Model file for the job. Use its own axes, mm. A direction names the side the tool comes from. Round coordinates to 2 decimals unless told otherwise and drop trailing zeros. Order: outer loops, then holes, each group sorted by start corner. A loop starts at its lowest first (then second) coordinate and runs counter-clockwise, first axis right, second up. Notation, with made-up numbers: M 85,-35.75 L 112,-35.75 A22 cw 112,2.25 Z; hole C 25.25,60 d4. An arc over 180 degrees is marked long. Return JSON: item names as keys, results as strings. Group by question number.
Item 1: Probe line 1 along Y through (x, z) = (-2.25, -8.75); line 2 along X through (y, z) = (-47.5, 1). List the from-to ranges inside material, lowest first.
Item 2: Which spindle directions (+Z, -Z, +X, -X, +Y, -Y) get a long thin tool onto all of the face, cutting with end or side? Do faces 4 (the face through (5, -49, 0.5)), 5 (the face through (0, 1, 0)), 6 (the face through (-2, -99.5, -2)), 7 (the face through (-5.78, 0.49, -7.54)), 8 (the face through (-0.5, -49, -5)). Say none if no direction does.
Item 3: Pin check, flat tips, straight feed: pin 1 Ø1.5 at (x, y) = (6, -42.5) entering from +Z; pin 2 Ø2.5 at (x, y) = (-6.5, -39.5) entering from -Z; pin 3 Ø8 at (y, z) = (-83, 8.5) entering from +X. Stop position of each tip, or through.
Item 4: Slice it at A-A on y = -38. Write the cut outline in (x, z).
Item 5: Slice it at B-B on z = 2.75. Write the cut outline in (x, y), then the cut area to 3 significant figures.
Item 6: Pull direction Y, two halves, no side cores. Call faces 1 (the face through (3.2, -100.2, -10)), 2 (the face through (0, -101, 0)), 3 (the face through (-5, -49, 0.5)): pulls with the +Y half, pulls with the -Y half, needs draft (parallel to the pull), parting line crosses it, or undercut.
from build123d import *

# Parameters (mm, degrees)
EXTRUDE_1_DEPTH          = 0.5
PATTERN_CIRCULAR_1_COUNT = 2
PATTERN_CIRCULAR_1_ANGLE = 90
SKETCH_3_R               = 9.5
EXTRUDE_2_DEPTH          = 1
SKETCH_4_R               = 10.5
EXTRUDE_3_DEPTH          = 1.5


with BuildPart() as part:
    # Эскиз1 → Бобышка-Вытянуть1 (new, symmetric)
    with BuildSketch(Plane.XY):
        with BuildLine():
            Line((-8.75, 0), (8.75, 0))
            Line((8.75, 0), (8.75, -12.322967039))
            ThreePointArc((8.75, -12.322967039), (8.57806723, -12.883595848), (8.121390676, -13.251443729))
            Line((8.121390676, -13.251443729), (3.75, -15))
            Line((3.75, -15), (8.121390676, -16.748556271))
            ThreePointArc((8.121390676, -16.748556271), (8.57806723, -17.116404152), (8.75, -17.677032961))
            Line((8.75, -17.677032961), (8.75, -78.763241336))
            ThreePointArc((8.75, -78.763241336), (8.395311893, -81.402930425), (7.356408303, -83.855366249))
            Line((7.356408303, -83.855366249), (6.593591697, -85.144633751))
            ThreePointArc((6.593591697, -85.144633751), (5.554688107, -87.597069575), (5.2, -90.236758664))
            Line((5.2, -90.236758664), (5.2, -99.5))
            Line((5.2, -99.5), (-5.2, -99.5))
            Line((-5.2, -99.5), (-5.2, -90.236758664))
            ThreePointArc((-5.2, -90.236758664), (-5.554688107, -87.597069575), (-6.593591697, -85.144633751))
            Line((-6.593591697, -85.144633751), (-7.356408303, -83.855366249))
            ThreePointArc((-7.356408303, -83.855366249), (-8.395311893, -81.402930425), (-8.75, -78.763241336))
            Line((-8.75, -78.763241336), (-8.75, -17.677032961))
            ThreePointArc((-8.75, -17.677032961), (-8.57806723, -17.116404152), (-8.121390676, -16.748556271))
            Line((-8.121390676, -16.748556271), (-3.75, -15))
            Line((-3.75, -15), (-8.121390676, -13.251443729))
            ThreePointArc((-8.121390676, -13.251443729), (-8.57806723, -12.883595848), (-8.75, -12.322967039))
            Line((-8.75, -12.322967039), (-8.75, 0))
        make_face()
    extrude_1 = extrude(amount=EXTRUDE_1_DEPTH, both=True)

    # Круговой массив1: Бобышка-Вытянуть1 ×2 about axis
    pattern_circular_1_axis = Axis((0, 0, 0), (0, 1, 0))
    for i in range(1, PATTERN_CIRCULAR_1_COUNT):
        add(extrude_1.rotate(pattern_circular_1_axis, i * PATTERN_CIRCULAR_1_ANGLE / (PATTERN_CIRCULAR_1_COUNT - 1)))

    # Эскиз3 → Бобышка-Вытянуть2 (add)
    with BuildSketch(Plane(origin=(0, 0, 0), x_dir=(1, 0, 0), z_dir=(0, 1, 0))):
        with Locations(Location((0, 0, 0), (0, 0, 270))):
            Circle(SKETCH_3_R)
    extrude(amount=EXTRUDE_2_DEPTH)

    # Эскиз4 → Бобышка-Вытянуть3 (add)
    with BuildSketch(Plane.XZ.offset(99.5)):
        with Locations(Location((0, 0, 0), (0, 0, 270))):
            Circle(SKETCH_4_R)
    extrude(amount=EXTRUDE_3_DEPTH)


solid = part.part
Output values:
{
 "1": {"line 1": "-101 to -99.5, 0 to 1", "line 2": "-0.5 to 0.5"},
 "2": {"face 4": "+Z, +X", "face 5": "+Z, -Z, +X, -X, +Y", "face 6": "none", "face 7": "+Y", "face 8": "-Z, -X"},
 "3": {"pin 1": "z = 0.5", "pin 2": "z = -0.5", "pin 3": "x = 0.5"},
 "4": {"outline": "M -8.75,-0.5 L -0.5,-0.5 L -0.5,-8.75 L 0.5,-8.75 L 0.5,-0.5 L 8.75,-0.5 L 8.75,0.5 L 0.5,0.5 L 0.5,8.75 L -0.5,8.75 L -0.5,0.5 L -8.75,0.5 Z"},
 "5": {"outline": "M -10.13,-101 L 10.13,-101 L 10.13,-99.5 L 0.5,-99.5 L 0.5,0 L 9.09,0 L 9.09,1 L -9.09,1 L -9.09,0 L -0.5,0 L -0.5,-99.5 L -10.13,-99.5 Z", "area": "148 mm²"},
 "6": {"face 1": "needs draft", "face 2": "pulls with the -Y half", "face 3": "undercut"}
}
